For this review, take the finished solid that the model builds, in its own axes (mm). Face numbers are marked on the shaded views. Give positions to 0.01 mm unless a question says otherwise; leave off trailing zeros. Loops run counter-clockwise (first coordinate to the right, second up) from the corner with the lowest first, then second, coordinate; pieces in that order, holes last. Notation, with made-up numbers: (61, 24) - (111, 24) arc R23 ccw to (111, 63) - close; hole circle Ø6 at (22.5, 69.5). An arc over 180 degrees is marked (long way). Answer as CSV lines item,"result".
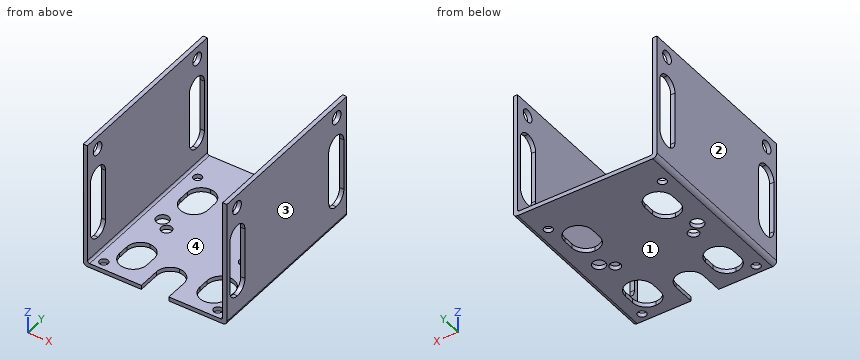
from build123d import *

# Parameters (mm, degrees)
F1_DEPTH  = 83
F3_DEPTH  = 68.001
F5_DEPTH  = 60.001
F6_R      = 3
F7_DEPTH  = 60.001
F8_R      = 2.5
F9_DEPTH  = 60.001
F10_R     = 2
F11_DEPTH = 60.001
F13_DEPTH = 60.001
F14_R     = 3
F15_DEPTH = 68.001


with BuildPart() as f1:
    # F0 (on Front) → F1 (new body)
    with BuildSketch(Plane.XZ):
        with BuildLine():
            ThreePointArc((0, 2), (0.585786, 0.585786), (2, 0))
            Line((2, 0), (66, 0))
            ThreePointArc((66, 0), (67.414214, 0.585786), (68, 2))
            Line((68, 2), (68, 60))
            Line((68, 60), (66, 60))
            Line((66, 60), (66, 3))
            ThreePointArc((66, 3), (65.707107, 2.292893), (65, 2))
            Line((65, 2), (3, 2))
            ThreePointArc((3, 2), (2.292893, 2.292893), (2, 3))
            Line((2, 3), (2, 60))
            Line((2, 60), (0, 60))
            Line((0, 60), (0, 2))
        make_face()
    extrude(amount=F1_DEPTH)

    # F2 (on face) → F3 (cut, through all)
    with BuildSketch(Plane.YZ.offset(68)):
        with BuildLine():
            Line((-81, 39.75), (-81, 15.25))
            ThreePointArc((-81, 15.25), (-79.462311, 11.537689), (-75.75, 10))
            ThreePointArc((-75.75, 10), (-72.037689, 11.537689), (-70.5, 15.25))
            Line((-70.5, 15.25), (-70.5, 39.75))
            ThreePointArc((-70.5, 39.75), (-72.037689, 43.462311), (-75.75, 45))
            ThreePointArc((-75.75, 45), (-79.462311, 43.462311), (-81, 39.75))
        make_face()
        with BuildLine():
            ThreePointArc((-7.25, 45), (-10.962311, 43.462311), (-12.5, 39.75))
            Line((-12.5, 39.75), (-12.5, 15.25))
            ThreePointArc((-12.5, 15.25), (-10.962311, 11.537689), (-7.25, 10))
            ThreePointArc((-7.25, 10), (-3.537689, 11.537689), (-2, 15.25))
            Line((-2, 15.25), (-2, 39.75))
            ThreePointArc((-2, 39.75), (-3.537689, 43.462311), (-7.25, 45))
        make_face()
    extrude(amount=-F3_DEPTH, mode=Mode.SUBTRACT)

    # F4 (on face) → F5 (cut, through all)
    with BuildSketch(Plane(origin=(0, 0, 0), x_dir=(1, 0, 0), z_dir=(0, 0, -1))):
        with BuildLine():
            Line((9, 71), (9, 66))
            ThreePointArc((9, 66), (10.903806, 61.403806), (15.5, 59.5))
            ThreePointArc((15.5, 59.5), (20.096194, 61.403806), (22, 66))
            Line((22, 66), (22, 71))
            ThreePointArc((22, 71), (20.096194, 75.596194), (15.5, 77.5))
            ThreePointArc((15.5, 77.5), (10.903806, 75.596194), (9, 71))
        make_face()
        with BuildLine():
            Line((60, 66), (60, 71))
            ThreePointArc((60, 71), (58.096194, 75.596194), (53.5, 77.5))
            ThreePointArc((53.5, 77.5), (48.903806, 75.596194), (47, 71))
            Line((47, 71), (47, 66))
            ThreePointArc((47, 66), (48.903806, 61.403806), (53.5, 59.5))
            ThreePointArc((53.5, 59.5), (58.096194, 61.403806), (60, 66))
        make_face()
        with BuildLine():
            Line((60, 24), (60, 29))
            ThreePointArc((60, 29), (58.096194, 33.596194), (53.5, 35.5))
            ThreePointArc((53.5, 35.5), (48.903806, 33.596194), (47, 29))
            Line((47, 29), (47, 24))
            ThreePointArc((47, 24), (48.903806, 19.403806), (53.5, 17.5))
            ThreePointArc((53.5, 17.5), (58.096194, 19.403806), (60, 24))
        make_face()
        with BuildLine():
            Line((22, 24), (22, 29))
            ThreePointArc((22, 29), (20.096194, 33.596194), (15.5, 35.5))
            ThreePointArc((15.5, 35.5), (10.903806, 33.596194), (9, 29))
            Line((9, 29), (9, 24))
            ThreePointArc((9, 24), (10.903806, 19.403806), (15.5, 17.5))
            ThreePointArc((15.5, 17.5), (20.096194, 19.403806), (22, 24))
        make_face()
    extrude(amount=-F5_DEPTH, mode=Mode.SUBTRACT)

    # F6 (on face) → F7 (cut, through all)
    with BuildSketch(Plane(origin=(0, 0, 0), x_dir=(1, 0, 0), z_dir=(0, 0, -1))):
        with Locations((57.25, 43.75)):
            Circle(F6_R)
        with Locations((10.75, 43.75)):
            Circle(F6_R)
    extrude(amount=-F7_DEPTH, mode=Mode.SUBTRACT)

    # F8 (on face) → F9 (cut, through all)
    with BuildSketch(Plane(origin=(0, 0, 0), x_dir=(1, 0, 0), z_dir=(0, 0, -1))):
        with Locations((15.5, 48)):
            Circle(F8_R)
        with Locations((52.5, 48)):
            Circle(F8_R)
    extrude(amount=-F9_DEPTH, mode=Mode.SUBTRACT)

    # F10 (on face) → F11 (cut, through all)
    with BuildSketch(Plane(origin=(0, 0, 0), x_dir=(1, 0, 0), z_dir=(0, 0, -1))):
        with Locations((7, 79)):
            Circle(F10_R)
        with Locations((61, 79)):
            Circle(F10_R)
        with Locations((7, 14)):
            Circle(F10_R)
        with Locations((61, 14)):
            Circle(F10_R)
    extrude(amount=-F11_DEPTH, mode=Mode.SUBTRACT)

    # F12 (on face) → F13 (cut, through all)
    with BuildSketch(Plane(origin=(0, 0, 0), x_dir=(1, 0, 0), z_dir=(0, 0, -1))):
        with BuildLine():
            Line((40.5, 83), (27.5, 83))
            Line((27.5, 83), (27.5, 72.5))
            ThreePointArc((27.5, 72.5), (29.403806, 67.903806), (34, 66))
            ThreePointArc((34, 66), (38.596194, 67.903806), (40.5, 72.5))
            Line((40.5, 72.5), (40.5, 83))
        make_face()
    extrude(amount=-F13_DEPTH, mode=Mode.SUBTRACT)

    # F14 (on face) → F15 (cut, through all)
    with BuildSketch(Plane(origin=(0, 0, 0), x_dir=(0, -1, 0), z_dir=(-1, 0, 0))):
        with Locations((7, 54)):
            Circle(F14_R)
        with Locations((76, 54)):
            Circle(F14_R)
    extrude(amount=-F15_DEPTH, mode=Mode.SUBTRACT)


solid = f1.part
1) Draft analysis for pull direction X (two halves, no side actions). For the marked faces 1, 2, 3 and 4, state which applies: pulls with the +X half, pulls with the -X half, needs draft (parallel to the pull), parting line crosses it, or undercut.
From the geometry:
face 1,"needs draft"
face 2,"pulls with the -X half"
face 3,"pulls with the +X half"
face 4,"undercut"
2) Consider section C-C on x = 48. Write out the cut boundary in (y, z).
From the geometry:
outline,"(-83, 0) - (-74.46, 0) - (-74.46, 2) - (-83, 2) - close; (-62.54, 0) - (-32.46, 0) - (-32.46, 2) - (-62.54, 2) - close; (-20.54, 0) - (0, 0) - (0, 2) - (-20.54, 2) - close"
3) Insertion check: P1, Ø0.6, axis at y = -67.5, z = 1, coming from the -X side; P2, Ø5.5, axis at x = 57.25, y = -43.75, coming from the +Z side; P3, Ø1.6, axis at y = -27.5, z = 1, coming from the -X side; P4, Ø8, axis at x = 57, y = -67.5, coming from the +Z side. Each pin has a flat end and moves straight along its axis. Give the tip position at first contact, or say it passes through.
From the geometry:
P1,"stops at x = 0.13"
P2,"passes through"
P3,"stops at x = 0.01"
P4,"stops at z = 2"
4) Consider section D-D on y = -14. Write out the cut boundary in (x, z), and give its area (3 significant figures).
From the geometry:
outline,"(0, 2) arc R2 ccw to (2, 0) - (5, 0) - (5, 2) - (3, 2) arc R1 cw to (2, 3) - (2, 60) - (0, 60) - close; (9, 0) - (59, 0) - (59, 2) - (9, 2) - close; (63, 0) - (66, 0) arc R2 ccw to (68, 2) - (68, 60) - (66, 60) - (66, 3) arc R1 cw to (65, 2) - (63, 2) - close"
area,"351 mm^2"
5) Wall thickness on line 1 (X direction, y = -40.5, z = 52); line 2 (Y direction, x = 52.5, z = 1.65); line 3 (Z direction, x = 67.45, y = -76): over which ranges is each line inside the solid? List them lowest first. Write a range as from..to.
From the geometry:
line 1,"x = 0..2, 66..68"
line 2,"y = -83..-77.42, -59.58..-50.5, -45.5..-35.42, -17.58..0"
line 3,"z = 0.62..10.01, 44.99..51, 57..60"
6) Consider section B-B on z = 54. Write out the cut boundary in (x, y).
From the geometry:
outline,"(0, -83) - (2, -83) - (2, -79) - (0, -79) - close; (0, -73) - (2, -73) - (2, -10) - (0, -10) - close; (0, -4) - (2, -4) - (2, 0) - (0, 0) - close; (66, -83) - (68, -83) - (68, -79) - (66, -79) - close; (66, -73) - (68, -73) - (68, -10) - (66, -10) - close; (66, -4) - (68, -4) - (68, 0) - (66, 0) - close"
7) Consider section A-A on y = -48. Write out the cut boundary in (x, z), and give its area (3 significant figures).
From the geometry:
outline,"(0, 2) arc R2 ccw to (2, 0) - (13, 0) - (13, 2) - (3, 2) arc R1 cw to (2, 3) - (2, 60) - (0, 60) - close; (18, 0) - (50, 0) - (50, 2) - (18, 2) - close; (55, 0) - (66, 0) arc R2 ccw to (68, 2) - (68, 60) - (66, 60) - (66, 3) arc R1 cw to (65, 2) - (55, 2) - close"
area,"347 mm^2"
